Geometry: final body of the model. Coordinates: model frame, mm. Give positions to 0.01 mm unless a question says otherwise; leave off trailing zeros. Write each loop counter-clockwise with the first axis right and the second up, starting at its lowest first coordinate (ties: lowest second). Pieces come first, ordered by that corner, then holes.
Q1. Cut plane B-B on x = 106. Count the separate pieces of the cut face and the enclosed holes in it, plus the area to 3 significant figures.
Q2. Cut plane A-A on y = -0.75. Return the cut outline in (x, z), plus the area to 3 significant figures.
Q3. Line query: L1, parallel to Y at x = 70, z = 1.25; L2, parallel to Y at x = 88, z = -9.75; L3, parallel to Z at x = 148.5, y = 12.3. Output: solid intervals per line, ascending.
Q4. Pin query (flat end, axial travel): pin 1 (1.6 mm diameter, centred on x = 74, z = -10.5, fed in from +Y); pin 2 (4.5 mm diameter, centred on x = 133.5, z = 0, fed in from +Y). Return the tip coordinate at first contact, or that it passes through.
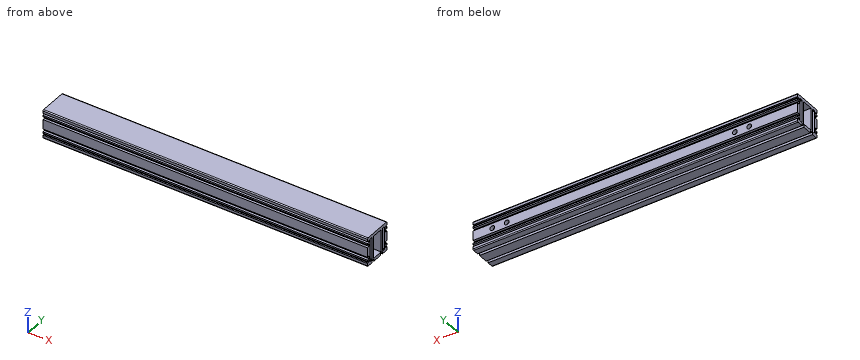
```python
from build123d import *

# Parameters (mm, degrees)
SKETCH_1_W             = 23.5
SKETCH_1_H             = 12
EXTRUDE_1_DEPTH        = 168.5
HOLE_WIZARD_M6_1_D     = 5
HOLE_WIZARD_M6_1_DEPTH = 15
HOLE_WIZARD_M6_1_TIP   = 1.502151548


with BuildPart() as part:
    # 草图1 → 凸台-拉伸1 (new, symmetric)
    with BuildSketch(Plane(origin=(0, 0, 0), x_dir=(0, 0, -1), z_dir=(1, 0, 0))):
        with BuildLine():
            Line((-14, 15), (-11.5, 15))
            Line((-11.5, 15), (-11.5, 13.5))
            Line((-11.5, 13.5), (-11.4, 13.5))
            ThreePointArc((-11.4, 13.5), (-11.117157288, 13.382842712), (-11, 13.1))
            Line((-11, 13.1), (-11, 12))
            Line((-11, 12), (-9.5, 12))
            Line((-9.5, 12), (-9.5, 15))
            Line((-9.5, 15), (-8, 15))
            Line((-8, 15), (-8, 12.5))
            Line((-8, 12.5), (-5, 12.5))
            Line((-5, 12.5), (-5, 15))
            Line((-5, 15), (5, 15))
            Line((5, 15), (5, 12.5))
            Line((5, 12.5), (8, 12.5))
            Line((8, 12.5), (8, 15))
            Line((8, 15), (9.5, 15))
            Line((9.5, 15), (9.5, 12))
            Line((9.5, 12), (11, 12))
            Line((11, 12), (11, 13.1))
            ThreePointArc((11, 13.1), (11.117157288, 13.382842712), (11.4, 13.5))
            Line((11.4, 13.5), (11.5, 13.5))
            Line((11.5, 13.5), (11.5, 15))
            Line((11.5, 15), (14, 15))
            ThreePointArc((14, 15), (14.707106781, 14.707106781), (15, 14))
            Line((15, 14), (15, 8))
            Line((15, 8), (12.5, 8))
            Line((12.5, 8), (12.5, 5))
            Line((12.5, 5), (15, 5))
            Line((15, 5), (15, -5))
            Line((15, -5), (12.5, -5))
            Line((12.5, -5), (12.5, -8))
            Line((12.5, -8), (15, -8))
            Line((15, -8), (15, -14))
            ThreePointArc((15, -14), (14.707106781, -14.707106781), (14, -15))
            Line((14, -15), (11.5, -15))
            Line((11.5, -15), (11.5, -13.5))
            Line((11.5, -13.5), (11.4, -13.5))
            ThreePointArc((11.4, -13.5), (11.117157288, -13.382842712), (11, -13.1))
            Line((11, -13.1), (11, -12))
            Line((11, -12), (9.5, -12))
            Line((9.5, -12), (9.5, -15))
            Line((9.5, -15), (8, -15))
            Line((8, -15), (8, -12.5))
            Line((8, -12.5), (5, -12.5))
            Line((5, -12.5), (5, -15))
            Line((5, -15), (-5, -15))
            Line((-5, -15), (-5, -12.5))
            Line((-5, -12.5), (-8, -12.5))
            Line((-8, -12.5), (-8, -15))
            Line((-8, -15), (-9.5, -15))
            Line((-9.5, -15), (-9.5, -12))
            Line((-9.5, -12), (-11, -12))
            Line((-11, -12), (-11, -13.1))
            ThreePointArc((-11, -13.1), (-11.117157288, -13.382842712), (-11.4, -13.5))
            Line((-11.4, -13.5), (-11.5, -13.5))
            Line((-11.5, -13.5), (-11.5, -15))
            Line((-11.5, -15), (-14, -15))
            ThreePointArc((-14, -15), (-14.707106781, -14.707106781), (-15, -14))
            Line((-15, -14), (-15, 14))
            ThreePointArc((-15, 14), (-14.707106781, 14.707106781), (-14, 15))
        make_face()
        with BuildLine():
            Line((12, -10.5), (12, -8.5))
            ThreePointArc((12, -8.5), (11.853553391, -8.146446609), (11.5, -8))
            Line((11.5, -8), (-11.5, -8))
            ThreePointArc((-11.5, -8), (-11.853553391, -8.146446609), (-12, -8.5))
            Line((-12, -8.5), (-12, -10.5))
            ThreePointArc((-12, -10.5), (-11.853553391, -10.853553391), (-11.5, -11))
            Line((-11.5, -11), (11.5, -11))
            ThreePointArc((11.5, -11), (11.853553391, -10.853553391), (12, -10.5))
        make_face(mode=Mode.SUBTRACT)
        with BuildLine():
            Line((-11.5, 11), (11.5, 11))
            ThreePointArc((11.5, 11), (11.853553391, 10.853553391), (12, 10.5))
            Line((12, 10.5), (12, 8.5))
            ThreePointArc((12, 8.5), (11.853553391, 8.146446609), (11.5, 8))
            Line((11.5, 8), (-11.5, 8))
            ThreePointArc((-11.5, 8), (-11.853553391, 8.146446609), (-12, 8.5))
            Line((-12, 8.5), (-12, 10.5))
            ThreePointArc((-12, 10.5), (-11.853553391, 10.853553391), (-11.5, 11))
        make_face(mode=Mode.SUBTRACT)
        Rectangle(SKETCH_1_W, SKETCH_1_H, mode=Mode.SUBTRACT)
    extrude(amount=EXTRUDE_1_DEPTH, both=True)

    # M6 螺纹孔1
    with Locations(Plane(origin=(0, 15, 0), x_dir=(-1, 0, 0), z_dir=(0, 1, 0))):
        with Locations((-148.5, 0), (-133.5, 0), (103.5, 0), (118.5, 0)):
            Hole(HOLE_WIZARD_M6_1_D / 2, depth=HOLE_WIZARD_M6_1_DEPTH)
            with Locations((0, 0, -(HOLE_WIZARD_M6_1_DEPTH + HOLE_WIZARD_M6_1_TIP / 2))):  # 118° drill point
                Cone(0, HOLE_WIZARD_M6_1_D / 2, HOLE_WIZARD_M6_1_TIP, mode=Mode.SUBTRACT)


solid = part.part
```
Data:
1. separate pieces: 1
1. enclosed holes: 3
1. area: 407 mm2
2. outline: (-168.5, -15) - (168.5, -15) - (168.5, -11.75) - (-168.5, -11.75) - close; (-168.5, 11.75) - (168.5, 11.75) - (168.5, 15) - (-168.5, 15) - close
2. area: 2,190 mm2
3. L1: y = -15 to -11, -8 to -6, 6 to 8, 11 to 15
3. L2: y = -12 to -11, -8 to -6, 6 to 8, 11 to 12
3. L3: z = -15 to -11, -9.5 to -2.5, 2.5 to 9.5, 11 to 15
4. pin 1: stops at y = 13.49
4. pin 2: stops at y = -6
